Could you check a few things on this model? Use its own coordinates, in mm. A direction names the side the tool comes from. Give positions to 0.01 mm unless a question says otherwise; leave off trailing zeros. Order: outer loops, then holes, each group sorted by start corner. A loop starts at its lowest first (then second) coordinate and runs counter-clockwise, first axis right, second up.
from build123d import *

# Parameters (mm, degrees)
BEARING_HOUSING_PROFILE_R          = 17
BEARING_HOUSING_PROFILE_R_2        = 11.1
BEARING_HOUSING_DEPTH              = 7
MOUNTING_WEB_PROFILE_W             = 42
MOUNTING_WEB_PROFILE_H             = 44
MOUNTING_WEB_DEPTH                 = 4
BEARING_SEAT_START                 = -50
BEARING_SEAT_PROFILE_R             = 11.1
BEARING_SEAT_DEPTH                 = 98.927027865
STANDOFF_FASTENERS_START           = -50
STANDOFF_FASTENERS_PROFILE_R       = 1.6
STANDOFF_FASTENERS_DEPTH           = 98.927027865
BEARING_KEEPER_FASTENERS_START     = -50
BEARING_KEEPER_FASTENERS_PROFILE_R = 1.1
BEARING_KEEPER_FASTENERS_DEPTH     = 98.927027865


with BuildPart() as part:
    # Bearing_housing_profile → Bearing_housing (new body)
    with BuildSketch(Plane.XY):
        Circle(BEARING_HOUSING_PROFILE_R)
        Circle(BEARING_HOUSING_PROFILE_R_2, mode=Mode.SUBTRACT)
    extrude(amount=BEARING_HOUSING_DEPTH)

    # Mounting_web_profile → Mounting_web (add)
    with BuildSketch(Plane.XY):
        with Locations((21, 0)):
            Rectangle(MOUNTING_WEB_PROFILE_W, MOUNTING_WEB_PROFILE_H)
    extrude(amount=MOUNTING_WEB_DEPTH)

    # Bearing_seat_profile → Bearing_seat (cut, through all)
    with BuildSketch(Plane.XY.offset(BEARING_SEAT_START)):
        Circle(BEARING_SEAT_PROFILE_R)
    extrude(amount=BEARING_SEAT_DEPTH, mode=Mode.SUBTRACT)

    # Standoff_fasteners_profile → Standoff_fasteners (cut, through all)
    with BuildSketch(Plane.XY.offset(STANDOFF_FASTENERS_START)):
        with Locations(Location((36, -18, 0), (0, 0, 180))):
            Circle(STANDOFF_FASTENERS_PROFILE_R)
        with Locations(Location((36, 18, 0), (0, 0, 180))):
            Circle(STANDOFF_FASTENERS_PROFILE_R)
    extrude(amount=STANDOFF_FASTENERS_DEPTH, mode=Mode.SUBTRACT)

    # Bearing_keeper_fasteners_profile → Bearing_keeper_fasteners (cut, through all)
    with BuildSketch(Plane.XY.offset(BEARING_KEEPER_FASTENERS_START)):
        with Locations(Location((-14, 0, 0), (0, 0, 180))):
            Circle(BEARING_KEEPER_FASTENERS_PROFILE_R)
        with Locations(Location((0, -14, 0), (0, 0, 180))):
            Circle(BEARING_KEEPER_FASTENERS_PROFILE_R)
        with Locations(Location((0, 14, 0), (0, 0, 180))):
            Circle(BEARING_KEEPER_FASTENERS_PROFILE_R)
    extrude(amount=BEARING_KEEPER_FASTENERS_DEPTH, mode=Mode.SUBTRACT)


solid = part.part
Item 1: For faces 1 (the flat face through (0, -20, 2)), 2 (the cylindrical face through (-16.984, 0.747, 4.229)), 3 (the flat face through (11, -4, 7)), which set-ups out of +Z, -Z, +X, -X, +Y, -Y let a thin tool reach every point of the face, with its end or its side?
Findings:
face 1: +Z, -Z, -X, -Y
face 2: +Z
face 3: +Z, +X, -X, +Y, -Y
Item 2: We'd pull the mould along X, two halves only. Please class faces 4 (the cylindrical face through (5.97, 9.36, 3.45)), 5 (the flat face through (0, 19, 2)), 6 (the flat face through (42, 0, 2)): +X half, -X half, draft (parallel to the pull), parting line (faces both ways), or undercut.
Findings:
face 4: undercut
face 5: -X half
face 6: +X half
Item 3: Imagine slicing it at B-B on z = 1.25. List the corners of the cut face in (x, y) for me.
Findings:
outline: (0, -22) - (42, -22) - (42, 22) - (0, 22) - (0, 17) arc R17 ccw to (0, -17) - close; hole circle Ø2.2 at (-14, 0); hole circle Ø22.2 at (0, 0); hole circle Ø2.2 at (0, -14); hole circle Ø2.2 at (0, 14); hole circle Ø3.2 at (36, -18); hole circle Ø3.2 at (36, 18)
Item 4: Please list where these lines run through material, in increasing order: line 1 along Y through (x, z) = (0, 4.5); line 2 along Y through (x, z) = (36, 3.1); line 3 along Y through (x, z) = (1, 4.75).
Findings:
line 1: y = -17 to -15.1, -12.9 to -11.1, 11.1 to 12.9, 15.1 to 17
line 2: y = -22 to -19.6, -16.4 to 16.4, 19.6 to 22
line 3: y = -16.97 to -14.46, -13.54 to -11.05, 11.05 to 13.54, 14.46 to 16.97
Item 5: Imagine slicing it at D-D on x = -6.5. List the corners of the cut face in (y, z) for me, then the cut area to 3 significant figures.
Findings:
outline: (-15.71, 0) - (-9, 0) - (-9, 7) - (-15.71, 7) - close; (9, 0) - (15.71, 0) - (15.71, 7) - (9, 7) - close
area: 93.9 mm2
Item 6: Imagine slicing it at A-A on y = 0. List the corners of the cut face in (x, z) for me.
Findings:
outline: (-17, 0) - (-15.1, 0) - (-15.1, 7) - (-17, 7) - close; (-12.9, 0) - (-11.1, 0) - (-11.1, 7) - (-12.9, 7) - close; (11.1, 0) - (42, 0) - (42, 4) - (17, 4) - (17, 7) - (11.1, 7) - close
Item 7: Imagine slicing it at C-C on y = -18. List the corners of the cut face in (x, z) for me.
Findings:
outline: (0, 0) - (34.4, 0) - (34.4, 4) - (0, 4) - close; (37.6, 0) - (42, 0) - (42, 4) - (37.6, 4) - close
Item 8: For pin 1 (3 mm diameter, centred on y = 20.5, z = 2, fed in from -X); pin 2 (5 mm diameter, centred on x = 36, y = 18, fed in from -Z); pin 3 (2 mm diameter, centred on x = -6.5, z = 2, fed in from -Y), each with a flat end and sliding along its axis, tell me the tip position at first contact or that it passes through.
Findings:
pin 1: stops at x = 0
pin 2: stops at z = 0
pin 3: stops at y = -16.09
